```python
from build123d import *

# Parameters (mm, degrees)
EXTRUDE_2_DEPTH     = 13
SKETCH_5_R          = 3.5
CUT_EXTRUDE_3_DEPTH = 13


with BuildPart() as part:
    # 草图1 → 凸台-拉伸2 (new body)
    with BuildSketch(Plane.XY):
        with BuildLine():
            Line((8.355798715, -13.336367576), (29.501926433, 27.06708322))
            ThreePointArc((29.501926433, 27.06708322), (29.0877743, 37.05850344), (20.227874503, 41.695547281))
            Line((20.227874503, 41.695547281), (-25.335604147, 39.806905679))
            ThreePointArc((-25.335604147, 39.806905679), (-33.78135181, 34.452529301), (-33.367199677, 24.461109081))
            Line((-33.367199677, 24.461109081), (-8.949848746, -14.053700113))
            ThreePointArc((-8.949848746, -14.053700113), (-0.089948949, -18.690743955), (8.355798715, -13.336367576))
        make_face()
    extrude(amount=EXTRUDE_2_DEPTH)

    # 草图5 → 切除-拉伸3 (cut)
    with BuildSketch(Plane.XY.offset(13)):
        with Locations((-0.945044174, 18.385896346)):
            Circle(SKETCH_5_R)
    extrude(amount=-CUT_EXTRUDE_3_DEPTH, mode=Mode.SUBTRACT)


solid = part.part
```
Check sheet for the modelled part. Datum: model origin and axes. Units: mm. Round coordinates to 2 decimals unless told otherwise and drop trailing zeros. Loops run counter-clockwise (first coordinate to the right, second up) from the corner with the lowest first, then second, coordinate; pieces in that order, holes last. Notation, with made-up numbers: (46.25, 87.25) -> (91.25, 87.25) arc R27 cw to (91.25, 109.25) -> close; hole circle Ø1 at (50, 48.25). An arc over 180 degrees is marked (long way). Answer in a Markdown table with one row per item.
Q1. Sectioned sample at D-D on y = -9.5. Enter the section's corners in (x, z).
Data:
| item | result |
|---|---|
| outline | (-11.84, 0) -> (10.36, 0) -> (10.36, 13) -> (-11.84, 13) -> close |
Q2. Sectioned sample at B-B on z = 1.5. Enter the section's corners in (x, y).
Data:
| item | result |
|---|---|
| outline | (-33.37, 24.46) -> (-8.95, -14.05) arc R10 ccw to (8.36, -13.34) -> (29.5, 27.07) arc R10 ccw to (20.23, 41.7) -> (-25.34, 39.81) arc R10 ccw to start; hole circle Ø7 at (-0.95, 18.39) |
Q3. Sectioned sample at C-C on x = -27.5. Enter the section's corners in (y, z), then the cut area to 3 significant figures.
Data:
| item | result |
|---|---|
| outline | (15.21, 0) -> (39.48, 0) -> (39.48, 13) -> (15.21, 13) -> close |
| area | 316 mm^2 |
Q4. Sectioned sample at A-A on y = 17. Enter the section's corners in (x, z).
Data:
| item | result |
|---|---|
| outline | (-28.64, 0) -> (-4.16, 0) -> (-4.16, 13) -> (-28.64, 13) -> close; (2.27, 0) -> (24.23, 0) -> (24.23, 13) -> (2.27, 13) -> close |
Q5. Thickness scan on L1, parallel to X at y = 18, z = 10.75; L2, parallel to X at y = 19, z = 5.5 (3 decimals); L3, parallel to Y at x = -2, z = 9.5. Record the ranges inside material, lowest first.
Data:
| item | result |
|---|---|
| L1 | x = -29.27 to -4.42, 2.53 to 24.76 |
| L2 | x = -29.905 to -4.391, 2.501 to 25.28 |
| L3 | y = -18.59 to 15.05, 21.72 to 40.77 |
Q6. Go/stop test with flat-tipped pins: P1, Ø2, axis at x = 14, z = 6, coming from the +Y side; P2, Ø1.5, axis at x = 7.5, z = 8.5, coming from the +Y side; P3, Ø4, axis at y = 21.5, z = 5.5, coming from the +X side (3 decimals); P4, Ø1, axis at x = 18, y = 0, coming from the -Z side. Record where each tip stops, or that it passes through.
Data:
| item | result |
|---|---|
| P1 | stops at y = 41.48 |
| P2 | stops at y = 41.2 |
| P3 | stops at x = 27.635 |
| P4 | passes through |
Q7. Release check for a two-part mould opening along X. For faces 1 (the face through (-21.329, 5.473, 6.409)), 2 (the face through (5, 19, 13)), 3 (the face through (-1.401, 21.856, 6.591)), 4 (the face through (19, 7, 6)) record: released by +X, released by -X, zero draft, split by the parting line, or undercut.
Data:
| item | result |
|---|---|
| face 1 | released by -X |
| face 2 | zero draft |
| face 3 | undercut |
| face 4 | released by +X |
